```python
from build123d import *

# Parameters (mm, degrees)
SKETCH1_W                 = 30
SKETCH1_H                 = 87
BOSS_EXTRUDE1_DEPTH       = 220
CUT_EXTRUDE1_DEPTH        = 239.472220604
SKETCH3_W                 = 22
SKETCH3_H                 = 22
CUT_EXTRUDE2_DEPTH        = 13
SKETCH4_W                 = 22
SKETCH4_H                 = 22
CUT_EXTRUDE3_DEPTH        = 13
CUT_EXTRUDE4_REACH        = 240.472
SKETCH5_W                 = 10
SKETCH5_H                 = 9
SKETCH6_W                 = 4
SKETCH6_H                 = 87
CUT_EXTRUDE5_DEPTH        = 197
F_4_0MM_DOWEL_HOLE1_D     = 4
F_4_0MM_DOWEL_HOLE1_DEPTH = 6
FILLET1_R                 = 2
FILLET2_R                 = 1


with BuildPart() as part:
    # Sketch1 → Boss-Extrude1 (new body)
    with BuildSketch(Plane.XY):
        with Locations((15, 43.5)):
            Rectangle(SKETCH1_W, SKETCH1_H)
    extrude(amount=BOSS_EXTRUDE1_DEPTH)

    # Sketch2 → Cut-Extrude1 (cut, through all)
    with BuildSketch(Plane(origin=(30, 0, 0), x_dir=(0, 0, -1), z_dir=(1, 0, 0))):
        Polygon((-192, 77), (-23, 77), (-6, 64), (0, 64), (0, 23), (-6, 23), (-23, 10), (-192, 10), (-208, 22), (-208, 65), align=None)
        Polygon((0, 87), (-12, 87), (0, 78), align=None)
        Polygon((0, 0), (-12, 0), (0, 9), align=None)
        Polygon((-220, 87), (-220, 72), (-200, 87), align=None)
        Polygon((-220, 0), (-220, 15), (-200, 0), align=None)
    extrude(amount=-CUT_EXTRUDE1_DEPTH, mode=Mode.SUBTRACT)

    # Sketch3 → Cut-Extrude2 (cut)
    with BuildSketch(Plane(origin=(0, 64, 0), x_dir=(-1, 0, 0), z_dir=(0, -1, 0))):
        with Locations((-15, -17)):
            Rectangle(SKETCH3_W, SKETCH3_H)
    extrude(amount=-CUT_EXTRUDE2_DEPTH, mode=Mode.SUBTRACT)

    # Sketch4 → Cut-Extrude3 (cut)
    with BuildSketch(Plane(origin=(0, 23, 0), x_dir=(1, 0, 0), z_dir=(0, 1, 0))):
        with Locations((15, -17)):
            Rectangle(SKETCH4_W, SKETCH4_H)
    extrude(amount=-CUT_EXTRUDE3_DEPTH, mode=Mode.SUBTRACT)

    # Sketch5 → Cut-Extrude4 (cut, up to next)
    with BuildSketch(Plane.XY.offset(220), mode=Mode.PRIVATE) as cut_extrude4_sk1:
        with Locations((15, 53.5)):
            Rectangle(SKETCH5_W, SKETCH5_H)
    cut_extrude4_tool1 = extrude(cut_extrude4_sk1.sketch, amount=-CUT_EXTRUDE4_REACH, mode=Mode.PRIVATE) & part.part
    # Sketch5 → Cut-Extrude4 (cut, up to next)
    with BuildSketch(Plane.XY.offset(220), mode=Mode.PRIVATE) as cut_extrude4_sk2:
        with Locations((15, 36.5)):
            Rectangle(SKETCH5_W, SKETCH5_H)
    cut_extrude4_tool2 = extrude(cut_extrude4_sk2.sketch, amount=-CUT_EXTRUDE4_REACH, mode=Mode.PRIVATE) & part.part
    add(cut_extrude4_tool1.solids().sort_by_distance((15, 53.5, 220))[0], mode=Mode.SUBTRACT)
    add(cut_extrude4_tool2.solids().sort_by_distance((15, 36.5, 220))[0], mode=Mode.SUBTRACT)

    # Sketch6 → Cut-Extrude5 (cut)
    with BuildSketch(Plane.XY.offset(220)):
        with Locations((2, 43.5)):
            Rectangle(SKETCH6_W, SKETCH6_H)
        with Locations((28, 43.5)):
            Rectangle(SKETCH6_W, SKETCH6_H)
    extrude(amount=-CUT_EXTRUDE5_DEPTH, mode=Mode.SUBTRACT)

    # Ø4.0mm Dowel Hole1
    with Locations(Plane.XY.offset(6)):
        with Locations((9, 16), (9, 71), (21, 71), (21, 16)):
            Hole(F_4_0MM_DOWEL_HOLE1_D / 2, depth=F_4_0MM_DOWEL_HOLE1_DEPTH)

    # Fillet1
    fillet1_edges = [part.edges().sort_by_distance(p)[0] for p in [
        (15, 49, 220),
        (15, 49, 208),
        (15, 41, 220),
        (15, 41, 208),
    ]]
    fillet(fillet1_edges, radius=FILLET1_R)

    # Fillet2
    # the kernel refuses this fillet: 1 mm, written as the material it adds along each edge
    with BuildSketch(Plane(origin=(10, 49, 218), x_dir=(1, 0, 0), z_dir=(0, 0, -1)), Plane(origin=(20, 41, 218), x_dir=(-1, 0, 0), z_dir=(0, 0, -1))) as fillet2_piece_1:
        with BuildLine():
            CenterArc((FILLET2_R, -FILLET2_R), FILLET2_R, 90, 90)
            Line((0, -FILLET2_R), (0, 0))
            Line((0, 0), (FILLET2_R, 0))
        make_face()
    extrude(amount=8)
    with BuildSketch(Plane(origin=(20, 49, 218), x_dir=(-1, 0, 0), z_dir=(0, 0, -1)), Plane(origin=(10, 41, 218), x_dir=(1, 0, 0), z_dir=(0, 0, -1))) as fillet2_piece_2:
        with BuildLine():
            CenterArc((FILLET2_R, FILLET2_R), FILLET2_R, 180, 90)
            Line((0, FILLET2_R), (0, 0))
            Line((0, 0), (FILLET2_R, 0))
        make_face()
    extrude(amount=8)
    with BuildSketch(Plane(origin=(10, 47, 210), x_dir=(0, -0.9491428341660849, -0.31484580408697216), z_dir=(0, -0.31484580408697216, 0.9491428341660849))) as fillet2_piece_3_section:
        with BuildLine():
            CenterArc((2 + FILLET2_R, FILLET2_R), FILLET2_R, 180, 90)
            Line((2 + FILLET2_R, 0), (2, 0))
            Line((2, 0), (2, FILLET2_R))
        make_face()
    fillet2_piece_3 = revolve(axis=Axis((10, 47, 210), (1, 0, 0)), revolution_arc=161.648494619, mode=Mode.PRIVATE)
    fillet2_piece_3 = split(fillet2_piece_3, bisect_by=Plane(origin=(10.272150961, 48.462196414, 208), z_dir=(0, 0, 1)), keep=Keep.TOP, mode=Mode.PRIVATE)
    add(fillet2_piece_3)
    with BuildSketch(Plane(origin=(20, 47, 210), x_dir=(0, -0.9491428341660849, -0.31484580408697216), z_dir=(0, -0.31484580408697216, 0.9491428341660849))) as fillet2_piece_4_section:
        with BuildLine():
            CenterArc((2 + FILLET2_R, -FILLET2_R), FILLET2_R, 90, 90)
            Line((2 + FILLET2_R, 0), (2, 0))
            Line((2, 0), (2, -FILLET2_R))
        make_face()
    fillet2_piece_4 = revolve(axis=Axis((20, 47, 210), (1, 0, 0)), revolution_arc=161.648494619, mode=Mode.PRIVATE)
    fillet2_piece_4 = split(fillet2_piece_4, bisect_by=Plane(origin=(19.727849107, 48.462196279, 208), z_dir=(0, 0, 1)), keep=Keep.TOP, mode=Mode.PRIVATE)
    add(fillet2_piece_4)
    with BuildSketch(Plane(origin=(20, 43, 210), x_dir=(0, 0.9491428341660849, -0.31484580408697216), z_dir=(0, 0.31484580408697216, 0.9491428341660849))) as fillet2_piece_5_section:
        with BuildLine():
            CenterArc((2 + FILLET2_R, FILLET2_R), FILLET2_R, 180, 90)
            Line((2 + FILLET2_R, 0), (2, 0))
            Line((2, 0), (2, FILLET2_R))
        make_face()
    fillet2_piece_5 = revolve(axis=Axis((20, 43, 210), (-1, 0, 0)), revolution_arc=161.648494619, mode=Mode.PRIVATE)
    fillet2_piece_5 = split(fillet2_piece_5, bisect_by=Plane(origin=(19.727848664, 41.537804063, 208), z_dir=(0, 0, 1)), keep=Keep.TOP, mode=Mode.PRIVATE)
    add(fillet2_piece_5)
    with BuildSketch(Plane(origin=(10, 43, 210), x_dir=(0, 0.9491428341660849, -0.31484580408697216), z_dir=(0, 0.31484580408697216, 0.9491428341660849))) as fillet2_piece_6_section:
        with BuildLine():
            CenterArc((2 + FILLET2_R, -FILLET2_R), FILLET2_R, 90, 90)
            Line((2 + FILLET2_R, 0), (2, 0))
            Line((2, 0), (2, -FILLET2_R))
        make_face()
    fillet2_piece_6 = revolve(axis=Axis((10, 43, 210), (-1, 0, 0)), revolution_arc=161.648494619, mode=Mode.PRIVATE)
    fillet2_piece_6 = split(fillet2_piece_6, bisect_by=Plane(origin=(10.272151404, 41.537803928, 208), z_dir=(0, 0, 1)), keep=Keep.TOP, mode=Mode.PRIVATE)
    add(fillet2_piece_6)
    with BuildSketch(Plane(origin=(20, 47, 218), x_dir=(0, -0.9491428341660849, 0.31484580408697216), z_dir=(0, -0.31484580408697216, -0.9491428341660849))) as fillet2_piece_7_section:
        with BuildLine():
            CenterArc((2 + FILLET2_R, FILLET2_R), FILLET2_R, 180, 90)
            Line((2 + FILLET2_R, 0), (2, 0))
            Line((2, 0), (2, FILLET2_R))
        make_face()
    fillet2_piece_7 = revolve(axis=Axis((20, 47, 218), (-1, 0, 0)), revolution_arc=161.648494619, mode=Mode.PRIVATE)
    fillet2_piece_7 = split(fillet2_piece_7, bisect_by=Plane(origin=(19.727849077, 48.462196209, 220), z_dir=(0, 0, -1)), keep=Keep.TOP, mode=Mode.PRIVATE)
    add(fillet2_piece_7)
    with BuildSketch(Plane(origin=(10, 47, 218), x_dir=(0, -0.9491428341660849, 0.31484580408697216), z_dir=(0, -0.31484580408697216, -0.9491428341660849))) as fillet2_piece_8_section:
        with BuildLine():
            CenterArc((2 + FILLET2_R, -FILLET2_R), FILLET2_R, 90, 90)
            Line((2, -FILLET2_R), (2, 0))
            Line((2, 0), (2 + FILLET2_R, 0))
        make_face()
    fillet2_piece_8 = revolve(axis=Axis((10, 47, 218), (-1, 0, 0)), revolution_arc=161.648494619, mode=Mode.PRIVATE)
    fillet2_piece_8 = split(fillet2_piece_8, bisect_by=Plane(origin=(10.272143952, 48.462199818, 220), z_dir=(0, 0, -1)), keep=Keep.TOP, mode=Mode.PRIVATE)
    add(fillet2_piece_8)
    with BuildSketch(Plane(origin=(10, 43, 218), x_dir=(0, 0.9491428341660849, 0.31484580408697216), z_dir=(0, 0.31484580408697216, -0.9491428341660849))) as fillet2_piece_9_section:
        with BuildLine():
            CenterArc((2 + FILLET2_R, FILLET2_R), FILLET2_R, 180, 90)
            Line((2 + FILLET2_R, 0), (2, 0))
            Line((2, 0), (2, FILLET2_R))
        make_face()
    fillet2_piece_9 = revolve(axis=Axis((10, 43, 218), (1, 0, 0)), revolution_arc=161.648494619, mode=Mode.PRIVATE)
    fillet2_piece_9 = split(fillet2_piece_9, bisect_by=Plane(origin=(10.272150964, 41.537803607, 220), z_dir=(0, 0, -1)), keep=Keep.TOP, mode=Mode.PRIVATE)
    add(fillet2_piece_9)
    with BuildSketch(Plane(origin=(20, 43, 218), x_dir=(0, 0.9491428341660849, 0.31484580408697216), z_dir=(0, 0.31484580408697216, -0.9491428341660849))) as fillet2_piece_10_section:
        with BuildLine():
            CenterArc((2 + FILLET2_R, -FILLET2_R), FILLET2_R, 90, 90)
            Line((2 + FILLET2_R, 0), (2, 0))
            Line((2, 0), (2, -FILLET2_R))
        make_face()
    fillet2_piece_10 = revolve(axis=Axis((20, 43, 218), (1, 0, 0)), revolution_arc=161.648494619, mode=Mode.PRIVATE)
    fillet2_piece_10 = split(fillet2_piece_10, bisect_by=Plane(origin=(19.727849077, 41.537803791, 220), z_dir=(0, 0, -1)), keep=Keep.TOP, mode=Mode.PRIVATE)
    add(fillet2_piece_10)
    # the kernel refuses this fillet: 1 mm, written as the material it takes off along each edge
    with BuildSketch(Plane(origin=(4, 0, 202.5), x_dir=(0, 1, 0), z_dir=(0, 0, -1)), Plane(origin=(26, 87, 202.5), x_dir=(0, -1, 0), z_dir=(0, 0, -1))) as fillet2_2_piece_1:
        with BuildLine():
            CenterArc((FILLET2_R, FILLET2_R), FILLET2_R, 180, 90)
            Line((0, FILLET2_R), (0, 0))
            Line((0, 0), (FILLET2_R, 0))
        make_face()
    extrude(amount=179.5, mode=Mode.SUBTRACT)
    with BuildSketch(Plane(origin=(4, 10, 23), x_dir=(0, -1, 0), z_dir=(0, 0, 1))) as fillet2_2_piece_2_section:
        with BuildLine():
            CenterArc((FILLET2_R, FILLET2_R), FILLET2_R, 180, 90)
            Line((0, FILLET2_R), (0, 0))
            Line((0, 0), (FILLET2_R, 0))
        make_face()
    fillet2_2_piece_2 = extrude(amount=171.5, mode=Mode.PRIVATE)
    fillet2_2_piece_2 = split(fillet2_2_piece_2, bisect_by=Plane(origin=(4.130770438, -71.137574021, 83.816567972), z_dir=(0, 0.8, -0.6)), keep=Keep.TOP, mode=Mode.PRIVATE)
    add(fillet2_2_piece_2, mode=Mode.SUBTRACT)
    with BuildSketch(Plane(origin=(4, 77, 194.5), x_dir=(0, 1, 0), z_dir=(0, 0, -1))) as fillet2_2_piece_3_section:
        with BuildLine():
            CenterArc((FILLET2_R, FILLET2_R), FILLET2_R, 180, 90)
            Line((0, FILLET2_R), (0, 0))
            Line((0, 0), (FILLET2_R, 0))
        make_face()
    fillet2_2_piece_3 = extrude(amount=171.5, mode=Mode.PRIVATE)
    fillet2_2_piece_3 = split(fillet2_2_piece_3, bisect_by=Plane(origin=(4.223692297, 117.641585147, 137.811219805), z_dir=(0, -0.8, -0.6)), keep=Keep.TOP, mode=Mode.PRIVATE)
    add(fillet2_2_piece_3, mode=Mode.SUBTRACT)
    with BuildSketch(Plane(origin=(4, 87, 202.5), x_dir=(0, -1, 0), z_dir=(0, 0, -1)), Plane(origin=(26, 0, 202.5), x_dir=(0, 1, 0), z_dir=(0, 0, -1))) as fillet2_2_piece_4:
        with BuildLine():
            CenterArc((FILLET2_R, -FILLET2_R), FILLET2_R, 90, 90)
            Line((0, -FILLET2_R), (0, 0))
            Line((0, 0), (FILLET2_R, 0))
        make_face()
    extrude(amount=179.5, mode=Mode.SUBTRACT)
    with BuildSketch(Plane(origin=(26, 10, 23), x_dir=(0, -1, 0), z_dir=(0, 0, 1))) as fillet2_2_piece_5_section:
        with BuildLine():
            CenterArc((FILLET2_R, -FILLET2_R), FILLET2_R, 90, 90)
            Line((0, -FILLET2_R), (0, 0))
            Line((0, 0), (FILLET2_R, 0))
        make_face()
    fillet2_2_piece_5 = extrude(amount=171.5, mode=Mode.PRIVATE)
    fillet2_2_piece_5 = split(fillet2_2_piece_5, bisect_by=Plane(origin=(25.869229562, -71.137574021, 83.816567972), z_dir=(0, 0.8, -0.6)), keep=Keep.TOP, mode=Mode.PRIVATE)
    add(fillet2_2_piece_5, mode=Mode.SUBTRACT)
    with BuildSketch(Plane(origin=(26, 77, 194.5), x_dir=(0, 1, 0), z_dir=(0, 0, -1))) as fillet2_2_piece_6_section:
        with BuildLine():
            CenterArc((FILLET2_R, -FILLET2_R), FILLET2_R, 90, 90)
            Line((0, -FILLET2_R), (0, 0))
            Line((0, 0), (FILLET2_R, 0))
        make_face()
    fillet2_2_piece_6 = extrude(amount=171.5, mode=Mode.PRIVATE)
    fillet2_2_piece_6 = split(fillet2_2_piece_6, bisect_by=Plane(origin=(25.776307703, 117.641585147, 137.811219805), z_dir=(0, -0.8, -0.6)), keep=Keep.TOP, mode=Mode.PRIVATE)
    add(fillet2_2_piece_6, mode=Mode.SUBTRACT)


solid = part.part
```
Model file for the job. Use its own axes, mm. A direction names the side the tool comes from. Round coordinates to 2 decimals unless told otherwise and drop trailing zeros. Write each loop counter-clockwise with the first axis right and the second up, starting at its lowest first coordinate (ties: lowest second). Pieces come first, ordered by that corner, then holes. Notation, with made-up numbers: (38, 36) -> (91, 36) arc R27 cw to (91, 70) -> close; hole circle Ø8 at (67.5, 64.5). An arc over 180 degrees is marked (long way). Answer as CSV lines item,"result".
1. Slice it at A-A, the plane x = 17. State how many separate pieces and enclosed holes the cut face has, plus the area to 3 significant figures.
Resolved:
separate pieces,"3"
enclosed holes,"0"
area,"4,920 mm²"
2. Mould opens along Y. For faces 1 (the face through (15.154, 79.395, 210.14)), 2 (the face through (15, 44, 220)), 3 (the face through (20, 54, 214)) say: +Y half, -Y half, draft (parallel to the pull), parting line (faces both ways), or undercut.
Resolved:
face 1,"+Y half"
face 2,"draft"
face 3,"undercut"
3. Slice it at B-B, the plane z = 90.5. List the corners of the cut face in (x, y), plus the area to 3 significant figures.
Resolved:
outline,"(4, 1) arc R1 ccw to (5, 0) -> (25, 0) arc R1 ccw to (26, 1) -> (26, 9) arc R1 ccw to (25, 10) -> (5, 10) arc R1 ccw to (4, 9) -> close; (4, 78) arc R1 ccw to (5, 77) -> (25, 77) arc R1 ccw to (26, 78) -> (26, 86) arc R1 ccw to (25, 87) -> (5, 87) arc R1 ccw to (4, 86) -> close"
area,"438 mm²"
4. Tool access for faces 4 (the face through (15.21, 82.56, 6.08)), 5 (the face through (4, 73, 11)), 6 (the face through (2.03, 16.59, 14.38)), 7 (the face through (15, 32, 214)), 8 (the face through (9, 18, 3)): list every direction of +Z, -Z, +X, -X, +Y, -Y with a clear straight run to the whole face (end or side of a thin tool).
Resolved:
face 4,"-Z, +X, -X, +Y"
face 5,"none"
face 6,"+Z, +X, -X"
face 7,"+Z, -Z"
face 8,"-Z"
5. Drill centre lines: line 1 (Y direction, x = 9, z = 4.25); line 2 (Z direction, x = 23.75, y = 16); line 3 (Y direction, x = 24, z = 164). Where is each one in solid material? Low to high.
Resolved:
line 1,"5.81 to 14, 18 to 23, 64 to 69, 73 to 81.19"
line 2,"0 to 6, 200 to 220"
line 3,"0 to 10, 77 to 87"
6. Pin check, flat tips, straight feed: pin 1 Ø2.5 at (y, z) = (37.5, 211.5) entering from +X; pin 2 Ø3 at (x, z) = (16, 214.5) entering from +Y; pin 3 Ø6.5 at (x, z) = (10, 100.5) entering from -Y; pin 4 Ø2.5 at (x, y) = (21, 16) entering from -Z. Stop position of each tip, or through.
Resolved:
pin 1,"x = 26"
pin 2,"y = 77.25"
pin 3,"y = 0"
pin 4,"z = 198.33"
7. Slice it at C-C, the plane y = 38. List the corners of the cut face in (x, z), plus the area to 3 significant figures.
Resolved:
outline,"(4, 208) -> (10, 208) -> (10, 220) -> (4, 220) -> close; (20, 208) -> (26, 208) -> (26, 220) -> (20, 220) -> close"
area,"144 mm²"
